Input: part model. Units: mm. Frame: model coordinates. A direction names the side the tool comes from. Coordinates: 2 decimals unless noted, no trailing zeros. Write each loop counter-clockwise with the first axis right and the second up, starting at its lowest first coordinate (ties: lowest second). Pieces come first, ordered by that corner, then holes. Notation, with made-up numbers: (22, 69) - (53, 69) arc R27 ccw to (53, 98) - close; hole circle Ø2 at (80, -16.75). An arc over 180 degrees is marked (long way). Use CSV: the item, a comma, the result in double quotes.
```python
from build123d import *

# Parameters (mm, degrees)
F0_W     = 50.588429
F0_H     = 38.504552
F0_W_2   = 21.09558
F0_H_2   = 16.999349
F1_DEPTH = 25
F2_W     = 27.401078
F2_H     = 13.22294
F3_DEPTH = 25
F4_W     = 10.518003
F4_H     = 9.934522
F5_DEPTH = 25


with BuildPart() as f1:
    # F0 (on Front) → F1 (new body)
    with BuildSketch(Plane.XZ):
        with Locations((-1.740897, 6.246749)):
            Rectangle(F0_W, F0_H)
        with Locations((-0.102405, 3.072171)):
            Rectangle(F0_W_2, F0_H_2, mode=Mode.SUBTRACT)
    extrude(amount=F1_DEPTH)

    # F2 (on face) → F3 (join)
    with BuildSketch(Plane.XY.offset(25.499025)):
        with Locations((-1.496977, -10.263078)):
            Rectangle(F2_W, F2_H)
    extrude(amount=F3_DEPTH)

    # F4 (on face) → F5 (join)
    with BuildSketch(Plane.YZ.offset(23.553317)):
        with Locations((-12.053044, 10.954987)):
            Rectangle(F4_W, F4_H)
    extrude(amount=F5_DEPTH)


solid = f1.part
```
(1) Cut plane C-C on y = -4.5. Return loops of the section in (x, z).
Check values:
outline,"(-27.04, -13.01) - (23.55, -13.01) - (23.55, 25.5) - (12.2, 25.5) - (12.2, 50.5) - (-15.2, 50.5) - (-15.2, 25.5) - (-27.04, 25.5) - close; hole (-10.65, -5.43) - (10.45, -5.43) - (10.45, 11.57) - (-10.65, 11.57) - close"
(2) Ray query, probe 1 along X at (y, z) = (-21.5, 8); probe 2 along Z at (x, y) = (8, -7.25); probe 3 along Z at (x, y) = (-8.5, -23). Return the intervals inside material, ascending. Write a range as from..to.
Check values:
probe 1,"-27.04..-10.65, 10.45..23.55"
probe 2,"-13.01..-5.43, 11.57..50.5"
probe 3,"-13.01..-5.43, 11.57..25.5"
(3) Cut plane B-B on x = -6.5. Return loops of the section in (y, z).
Check values:
outline,"(-25, -13.01) - (0, -13.01) - (0, -5.43) - (-25, -5.43) - close; (-25, 11.57) - (0, 11.57) - (0, 25.5) - (-3.65, 25.5) - (-3.65, 50.5) - (-16.87, 50.5) - (-16.87, 25.5) - (-25, 25.5) - close"
(4) Cut plane A-A on y = -22.75. Return loops of the section in (x, z).
Check values:
outline,"(-27.04, -13.01) - (23.55, -13.01) - (23.55, 25.5) - (-27.04, 25.5) - close; hole (-10.65, -5.43) - (10.45, -5.43) - (10.45, 11.57) - (-10.65, 11.57) - close"
(5) Draft query along X for faces 4 (the flat face through (36, -12, 15.922)), 5 (the flat face through (12.204, -10, 38)), 6 (the flat face through (10.445, -12, 3)). Return one class per face: pulls with the +X half, pulls with the -X half, needs draft (parallel to the pull), parting line crosses it, or undercut.
Check values:
face 4,"needs draft"
face 5,"pulls with the +X half"
face 6,"undercut"
(6) Reachability of faces 1 (the flat face through (-15.198, -10, 38)), 2 (the flat face through (-2, -16.875, 38)), 3 (the flat face through (36, -12, 5.988)) from +Z, -Z, +X, -X, +Y, -Y: full face, straight path, thin tool, end or side. Return the list, or none.
Check values:
face 1,"+Z, -X, +Y, -Y"
face 2,"+Z, +X, -X, -Y"
face 3,"-Z, +X, +Y, -Y"
(7) Pin query (flat end, axial travel): pin 1 Ø11.5 at (x, y) = (37, -10) entering from -Z; pin 2 Ø12.5 at (x, z) = (-1.5, 36.5) entering from -Y; pin 3 Ø10.5 at (y, z) = (-7.5, 37.5) entering from +X. Return the tip coordinate at first contact, or that it passes through.
Check values:
pin 1,"z = 5.99"
pin 2,"y = -16.87"
pin 3,"x = 12.2"
(8) Cut plane D-D on z = 46. Return loops of the section in (x, y).
Check values:
outline,"(-15.2, -16.87) - (12.2, -16.87) - (12.2, -3.65) - (-15.2, -3.65) - close"
